Can you work these out from the model? Positions are in its coordinate system, mm. Coordinates: 2 decimals unless noted, no trailing zeros. Order: outer loops, then holes, each group sorted by start corner. A loop starts at its lowest first (then second) coordinate and runs counter-clockwise, first axis right, second up.
```python
from build123d import *

# Parameters (mm, degrees)
SKETCH_1_W          = 40
SKETCH_1_H          = 70
SKETCH_1_R          = 11
EXTRUDE_1_DEPTH     = 6
SKETCH_2_R          = 2
CUT_EXTRUDE_1_DEPTH = 10


with BuildPart() as part:
    # 草图1 → 凸台-拉伸1 (new body)
    with BuildSketch(Plane.XY):
        with Locations((-20, 79.503169777)):
            Rectangle(SKETCH_1_W, SKETCH_1_H)
        with Locations((-20, 79.503169777)):
            Circle(SKETCH_1_R, mode=Mode.SUBTRACT)
    extrude(amount=EXTRUDE_1_DEPTH)

    # 草图2 → 切除-拉伸1 (cut)
    with BuildSketch(Plane.XY.offset(6)):
        with Locations((-32, 104.503169777)):
            Circle(SKETCH_2_R)
        with Locations((-8, 104.503169777)):
            Circle(SKETCH_2_R)
    cut_extrude_1 = extrude(amount=-CUT_EXTRUDE_1_DEPTH, mode=Mode.SUBTRACT)

    # 镜向1: 切除-拉伸1 across plane
    add(cut_extrude_1.mirror(Plane.ZX.offset(79.503169777)), mode=Mode.SUBTRACT)


solid = part.part
```
1. Imagine slicing it at A-A on x = -20. Please give me the cut outline in (y, z).
Completed:
outline: (44.5, 0) - (68.5, 0) - (68.5, 6) - (44.5, 6) - close; (90.5, 0) - (114.5, 0) - (114.5, 6) - (90.5, 6) - close
2. Please list where these lines run through material, in increasing order: probe 1 along Y at (x, z) = (-8, 1.3); probe 2 along Y at (x, z) = (-20, 4.35); probe 3 along X at (y, z) = (106, 3.35).
Completed:
probe 1: y = 44.5 to 52.5, 56.5 to 102.5, 106.5 to 114.5
probe 2: y = 44.5 to 68.5, 90.5 to 114.5
probe 3: x = -40 to -33.33, -30.67 to -9.33, -6.67 to 0
3. Thinking about a two-plate mould opening in X: for faces 1 (the flat face through (-40, 79, 3)), 2 (the cylindrical face through (-30.925, 106.19, 3.042)), 3 (the flat face through (-11, 72, 0)), which applies, pulls with the +X half, pulls with the -X half, needs draft (parallel to the pull), parting line crosses it, or undercut?
Completed:
face 1: pulls with the -X half
face 2: undercut
face 3: needs draft
4. Imagine slicing it at C-C on y = 76. Please give me the cut outline in (x, z), then the cut area to 3 significant figures.
Completed:
outline: (-40, 0) - (-30.43, 0) - (-30.43, 6) - (-40, 6) - close; (-9.57, 0) - (0, 0) - (0, 6) - (-9.57, 6) - close
area: 115 mm2
5. Imagine slicing it at D-D on z = 3.3. Please give me the cut outline in (x, y), then the cut area to 3 significant figures.
Completed:
outline: (-40, 44.5) - (0, 44.5) - (0, 114.5) - (-40, 114.5) - close; hole circle Ø4 at (-32, 54.5); hole circle Ø4 at (-32, 104.5); hole circle Ø22 at (-20, 79.5); hole circle Ø4 at (-8, 54.5); hole circle Ø4 at (-8, 104.5)
area: 2,370 mm2
6. I'm going to push flat-ended pins straight in: pin 1 (17.5 mm diameter, centred on x = -20, y = 79.5, fed in from +Z); pin 2 (5 mm diameter, centred on x = -8, y = 104.5, fed in from -Z). Where does each tip first touch, or does it pass through?
Completed:
pin 1: passes through
pin 2: stops at z = 0
7. Imagine slicing it at B-B on x = -8. Please give me the cut outline in (y, z), then the cut area to 3 significant figures.
Completed:
outline: (44.5, 0) - (52.5, 0) - (52.5, 6) - (44.5, 6) - close; (56.5, 0) - (102.5, 0) - (102.5, 6) - (56.5, 6) - close; (106.5, 0) - (114.5, 0) - (114.5, 6) - (106.5, 6) - close
area: 372 mm2
